CAD build for the part. Positions are in the model's coordinates, mm. Give positions to 0.01 mm unless a question says otherwise; leave off trailing zeros. Write each loop counter-clockwise with the first axis right and the second up, starting at its lowest first coordinate (ties: lowest second). Pieces come first, ordered by that corner, then holes. Notation, with made-up numbers: (65, 4.5) - (102, 4.5) arc R21 ccw to (102, 29.5) - close; hole circle Ø8 at (53, 74.25). An arc over 180 degrees is marked (long way). Put each result on its own line as item: value. Start each with the question number.
1. Wall check: line 1 (Y direction, x = 1, z = 3.75); line 2 (X direction, y = 50, z = 4.1); line 3 (Y direction, x = -24.5, z = 0.4). Give the ranges that are in metal, low to high.
2. Cut at A-A on z = 1.75. List the corners of the cut face in (x, y).
3. Drop flat-ended pins along their axis: pin 1 (10 mm diameter, centred on x = -19.5, y = 20, fed in from +Z); pin 2 (2.5 mm diameter, centred on x = -52.5, z = 2, fed in from +Y). Give the stop position or say it passes through.
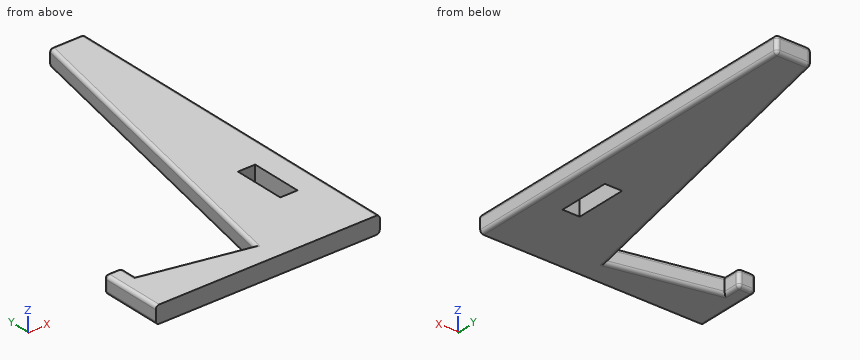
from build123d import *

# Parameters (mm, degrees)
SKETCH_W      = 5
SKETCH_H      = 15
EXTRUDE_DEPTH = 5
FILLET_R      = 1


with BuildPart() as part:
    # Sketch → Extrude (new body)
    with BuildSketch(Plane.XY):
        Polygon((10, 77.5), (10, -27.5), (-55, -27.5), (-55, -9.151514), (-50, -9.151514), (-50, -14.151514), (-20.646372, -20.345426), (0, 77.5), align=None)
        Rectangle(SKETCH_W, SKETCH_H, mode=Mode.SUBTRACT)
    extrude(amount=EXTRUDE_DEPTH)

    # Fillet
    fillet_edges = [part.edges().sort_by_distance(p)[0] for p in [
        (10, 77.5, 2.5),
        (10, 25, 0),
        (10, 25, 5),
        (-55, -9.151514, 2.5),
        (-55, -18.325757, 0),
        (-55, -18.325757, 5),
        (-50, -9.151514, 2.5),
        (-52.5, -9.151514, 0),
        (-52.5, -9.151514, 5),
        (-50, -11.651514, 0),
        (-50, -11.651514, 5),
        (-35.323186, -17.24847, 0),
        (-35.323186, -17.24847, 5),
        (0, 77.5, 2.5),
        (-10.323186, 28.577287, 0),
        (-10.323186, 28.577287, 5),
        (5, 77.5, 0),
        (5, 77.5, 5),
    ]]
    fillet(fillet_edges, radius=FILLET_R)


solid = part.part
Report:
1. line 1: y = -27.5 to -7.5, 7.5 to 77.5
1. line 2: x = -5.8 to 9.99
1. line 3: y = -27.5 to -19.74
2. outline: (-55, -27.5) - (10, -27.5) - (10, 76.5) arc R1 ccw to (9, 77.5) - (0.81, 77.5) arc R1 ccw to (-0.17, 76.71) - (-20.65, -20.35) - (-50, -14.15) - (-50, -10.15) arc R1 ccw to (-51, -9.15) - (-54, -9.15) arc R1 ccw to (-55, -10.15) - close; hole (-2.5, -7.5) - (2.5, -7.5) - (2.5, 7.5) - (-2.5, 7.5) - close
3. pin 1: passes through
3. pin 2: stops at y = -9.15
